```python
from build123d import *

# Parameters (mm, degrees)
SKIZZE1_R                            = 18.5
SKIZZE1_R_2                          = 10.65
AUFSATZ_LINEAR_AUSTRAGEN1_DEPTH      = 88.2
SKIZZE2_W                            = 10
SKIZZE2_H                            = 10
SCHNITT_LINEAR_AUSTRAGEN1_DEPTH      = 19.5
SCHNITT_LINEAR_AUSTRAGEN1_DEPTH_BACK = 19.5


with BuildPart() as part:
    # Skizze1 → Aufsatz-Linear austragen1 (new body)
    with BuildSketch(Plane.XY):
        Circle(SKIZZE1_R)
        Circle(SKIZZE1_R_2, mode=Mode.SUBTRACT)
    extrude(amount=AUFSATZ_LINEAR_AUSTRAGEN1_DEPTH)

    # Skizze2 → Schnitt-Linear austragen1 (cut, two sides)
    with BuildSketch(Plane(origin=(0, 0, 0), x_dir=(0, 0, -1), z_dir=(1, 0, 0))) as schnitt_linear_austragen1_sk:
        with Locations((-20, 13.5)):
            Rectangle(SKIZZE2_W, SKIZZE2_H)
    extrude(amount=SCHNITT_LINEAR_AUSTRAGEN1_DEPTH, mode=Mode.SUBTRACT)
    extrude(schnitt_linear_austragen1_sk.sketch, amount=-SCHNITT_LINEAR_AUSTRAGEN1_DEPTH_BACK, mode=Mode.SUBTRACT)


solid = part.part
```
Geometry check sheet. Reference: the model listing, model coordinates, mm. A direction names the side the tool comes from. Give positions to 0.01 mm unless a question says otherwise; leave off trailing zeros. Order: outer loops, then holes, each group sorted by start corner. A loop starts at its lowest first (then second) coordinate and runs counter-clockwise, first axis right, second up. Notation, with made-up numbers: (37.25, 22.5) - (42.25, 22.5) arc R17 cw to (42.25, 32.5) - close; hole circle Ø10 at (41.25, 9.25). An arc over 180 degrees is marked (long way). Write item = value, one per line. Start each with the question number.
1) Access from +Z, -Z, +X, -X, +Y, -Y to the whole of each face (thin tool, end or side, straight path). Record for faces 5 (the flat face through (0, 13, 25)), 6 (the flat face through (8, -8, 88.2)).
2) Section check C-C (x = 0). Enter the section's corners in (y, z), then the cut area to 3 significant figures.
3) Scan lines: L1, parallel to Z at x = -12, y = 12; L2, parallel to Y at x = 0, z = 33; L3, parallel to X at y = -0.5, z = 41.5. Record each from-to range of solid material in increasing order.
4) Draft check along Y on faces 1 (the cylindrical face through (-2.3, -10.4, 43.5)), 2 (the flat face through (8, -8, 0)), 3 (the flat face through (-11, 8.5, 20)), 4 (the cylindrical face through (-4.01, -18.06, 43.48)). Enter one of: released by +Y, released by -Y, zero draft, split by the parting line, or undercut.
5) Section check A-A (x = 8.5). Enter the section's corners in (y, z).
6) Section check D-D (z = 31). Enter the section's corners in (x, y).
7) Gauge pin test, flat ends, axial feed: pin 1 Ø2 at (x, y) = (8, 1.5) entering from +Z; pin 2 Ø6 at (x, z) = (-11.5, 76.5) entering from +Y; pin 3 Ø1.5 at (x, z) = (-5, 47) entering from +Y; pin 4 Ø8 at (x, z) = (12.5, 22.5) entering from +Y. Record the tip position at first contact, or that the pin passes through.
8) Section check B-B (y = 0). Enter the section's corners in (x, z), then the cut area to 3 significant figures.
Geometry check:
q1.face_5 = +X, -X, +Y
q1.face_6 = +Z, +X, -X, +Y, -Y
q2.outline = (-18.5, 0) - (-10.65, 0) - (-10.65, 88.2) - (-18.5, 88.2) - close; (10.65, 0) - (18.5, 0) - (18.5, 15) - (10.65, 15) - close; (10.65, 25) - (18.5, 25) - (18.5, 88.2) - (10.65, 88.2) - close
q2.area = 1,310 mm2
q3.L1 = 0 to 15, 25 to 88.2
q3.L2 = -18.5 to -10.65, 10.65 to 18.5
q3.L3 = -18.49 to -10.64, 10.64 to 18.49
q4.face_1 = undercut
q4.face_2 = zero draft
q4.face_3 = released by +Y
q4.face_4 = split by the parting line
q5.outline = (-16.43, 0) - (-6.42, 0) - (-6.42, 88.2) - (-16.43, 88.2) - close; (6.42, 0) - (16.43, 0) - (16.43, 15) - (8.5, 15) - (8.5, 25) - (16.43, 25) - (16.43, 88.2) - (6.42, 88.2) - close
q6.outline = circle Ø37 at (0, 0); hole circle Ø21.3 at (0, 0)
q7.pin_1 = through
q7.pin_2 = 16.43
q7.pin_3 = 18.01
q7.pin_4 = 15.95
q8.outline = (-18.5, 0) - (-10.65, 0) - (-10.65, 88.2) - (-18.5, 88.2) - close; (10.65, 0) - (18.5, 0) - (18.5, 88.2) - (10.65, 88.2) - close
q8.area = 1,380 mm2
